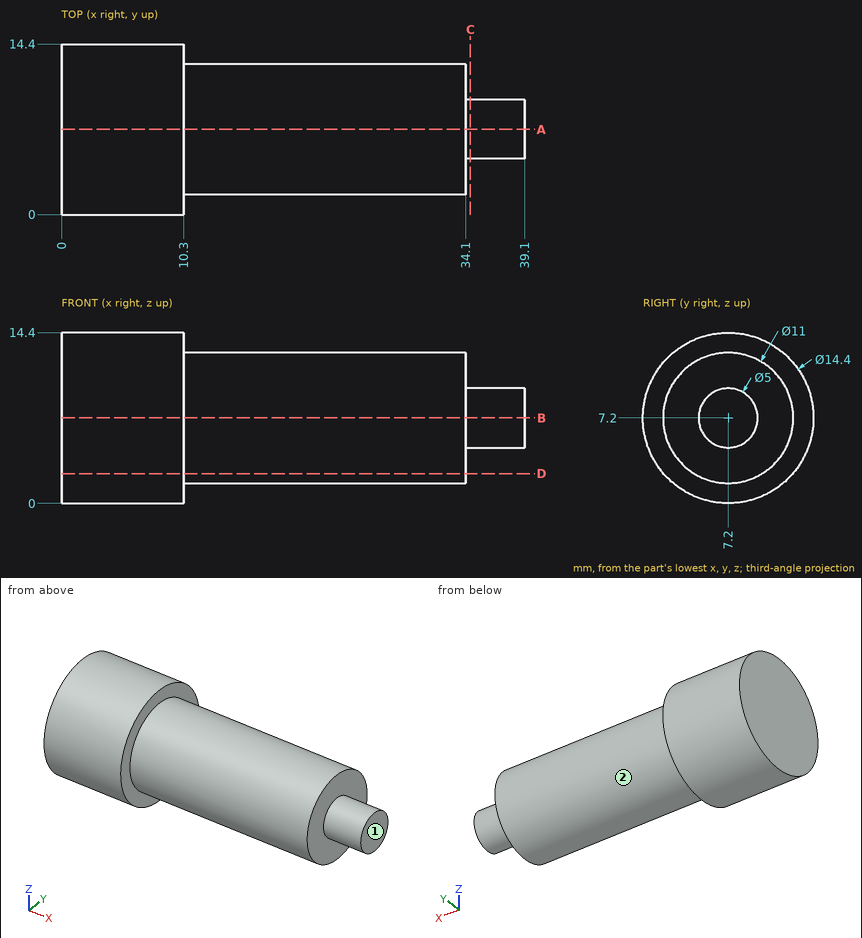
Could you check a few things on this drawing? It's one solid part, dimensions in mm from its lowest x, y, z. A direction names the side the tool comes from. Round coordinates to 2 decimals unless told otherwise and drop trailing zeros. Write each loop counter-clockwise with the first axis right and the second up, starting at its lowest first coordinate (ties: lowest second). Pieces come first, ordered by that corner, then holes.
Q1. If we section it at C-C on x = 34.5: Write out the boundary of the cut face in (y, z), plus the area to 3 significant figures.
Q2. Please list where these lines run through material, in increasing order: probe 1 along X at (y, z) = (1.75, 8.5); probe 2 along X at (y, z) = (9, 3); probe 3 along Z at (x, y) = (8, 12.5).
Q3. If we section it at A-A on y = 7.2: Write out the boundary of the cut face in (x, z).
Q4. Will these pins go through, and if not, where does the flat tip stop? P1, Ø2, axis at x = 6, z = 4.5, coming from the +Y side; P2, Ø4, axis at x = 4.5, y = 10, coming from the +Z side; P3, Ø1, axis at x = 6, z = 5.5, coming from the +Y side.
Q5. Which directions (+Z, -Z, +X, -X, +Y, -Y) give clear straight access to the entire face, cutting with the end or side of a thin tool? Please do the marked faces 1 and 2.
Q6. If we section it at D-D on z = 2.5: Write out the boundary of the cut face in (x, y).
Answer below:
1. outline: circle Ø5 at (7.2, 7.2)
1. area: 19.6 mm2
2. probe 1: x = 0 to 10.3
2. probe 2: x = 0 to 34.1
2. probe 3: z = 2.33 to 12.07
3. outline: (0, 0) - (10.3, 0) - (10.3, 1.7) - (34.1, 1.7) - (34.1, 4.7) - (39.1, 4.7) - (39.1, 9.7) - (34.1, 9.7) - (34.1, 12.7) - (10.3, 12.7) - (10.3, 14.4) - (0, 14.4) - close
4. P1: stops at y = 14.2
4. P2: stops at z = 14.36
4. P3: stops at y = 14.3
5. face 1: +Z, -Z, +X, +Y, -Y
5. face 2: +X
6. outline: (0, 1.75) - (10.3, 1.75) - (10.3, 4.34) - (34.1, 4.34) - (34.1, 10.06) - (10.3, 10.06) - (10.3, 12.65) - (0, 12.65) - close
